Drawing for the job (mm, zero at the part's lowest x, y, z). Coordinates: 2 decimals unless noted, no trailing zeros. Loops run counter-clockwise (first coordinate to the right, second up) from the corner with the lowest first, then second, coordinate; pieces in that order, holes last. Notation, with made-up numbers: (-19.5, 48) -> (21.5, 48) arc R26 cw to (21.5, 70) -> close; hole circle Ø8 at (-18, -30.5). An arc over 180 degrees is marked (long way). Write item = value, one per line. Start each with the question number.
(1) Band-saw the part on A-A (x = 299). Write the cut outline in (y, z), and give its area (3 significant figures).
(2) Band-saw the part on B-B (z = 28). Write the cut outline in (x, y) (3 decimals), and give its area (3 significant figures).
(3) Pull direction Y, two halves, no side cores. Call the marked faces 1 and 2: +Y half, -Y half, draft (parallel to the pull), parting line (faces both ways), or undercut.
(4) Flat gauge pins, fed straight in: P1, Ø1.9, axis at x = 232.5, y = 16.5, coming from the +Z side; P2, Ø9.5, axis at x = 449, z = 38, coming from the +Y side (3 decimals); P3, Ø3, axis at y = 15, z = 19, coming from the -X side. Where does each tip first touch, or does it go through?
(5) Band-saw the part on C-C (z = 51.5). Write the cut outline in (x, y) (3 decimals).
(6) Drill centre lines: line 1 (Y direction, x = 300.5, z = 40.5); line 2 (Z direction, x = 54, y = 14.25); line 3 (X direction, y = 13.25, z = 13) (3 decimals). Where is each one in solid material? Low to high. Write a range as from..to.
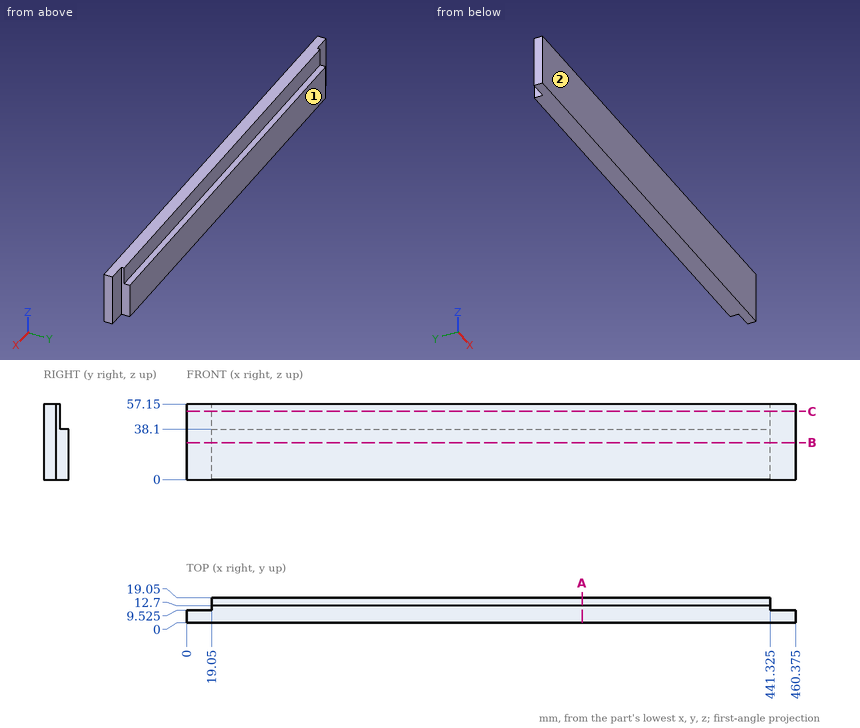
Findings below:
q1.outline = (0, 0) -> (19.05, 0) -> (19.05, 38.1) -> (12.7, 38.1) -> (12.7, 57.15) -> (0, 57.15) -> close
q1.area = 968 mm²
q2.outline = (0, 0) -> (460.375, 0) -> (460.375, 9.525) -> (441.325, 9.525) -> (441.325, 19.05) -> (19.05, 19.05) -> (19.05, 9.525) -> (0, 9.525) -> close
q2.area = 8,410 mm²
q3.face_1 = +Y half
q3.face_2 = -Y half
q4.P1 = 38.1
q4.P2 = 9.525
q4.P3 = 19.05
q5.outline = (0, 0) -> (460.375, 0) -> (460.375, 9.525) -> (441.325, 9.525) -> (441.325, 12.7) -> (19.05, 12.7) -> (19.05, 9.525) -> (0, 9.525) -> close
q6.line_1 = 0..12.7
q6.line_2 = 0..38.1
q6.line_3 = 19.05..441.325
